Can you work these out from the model? Positions are in its coordinate system, mm. Face numbers are marked on the shaded views. A direction names the side the tool comes from. Round coordinates to 2 decimals unless told otherwise and drop trailing zeros. Loops run counter-clockwise (first coordinate to the right, second up) from the corner with the lowest first, then second, coordinate; pieces in that order, holes last. Notation, with made-up numbers: M 66.5,-24 L 88.5,-24 A23 ccw 88.5,14 Z; hole C -9.5,36.25 d4. An arc over 180 degrees is marked long. Answer as CSV lines item,"result".
from build123d import *

# Parameters (mm, degrees)
SKETCH1_R           = 2.75
BOSS_EXTRUDE1_DEPTH = 30
CUT_EXTRUDE1_DEPTH  = 27
SKETCH4_3_R         = 6
CUT_EXTRUDE2_DEPTH  = 27


with BuildPart() as part:
    # Sketch1 → Boss-Extrude1 (new body)
    with BuildSketch(Plane(origin=(0, 0, 0), x_dir=(1, 0, 0), z_dir=(0, 1, 0))):
        with BuildLine():
            Line((42, 10.085339835), (-42, 10.085339835))
            ThreePointArc((-42, 10.085339835), (-52.085339835, 0), (-42, -10.085339835))
            Line((-42, -10.085339835), (42, -10.085339835))
            ThreePointArc((42, -10.085339835), (52.085339835, 0), (42, 10.085339835))
        make_face()
        with Locations((-42, 0)):
            Circle(SKETCH1_R, mode=Mode.SUBTRACT)
        with Locations((42, 0)):
            Circle(SKETCH1_R, mode=Mode.SUBTRACT)
    extrude(amount=BOSS_EXTRUDE1_DEPTH)

    # Sketch4 → Cut-Extrude1 (cut)
    with BuildSketch(Plane(origin=(0, 0, -10.085339835), x_dir=(-1, 0, 0), z_dir=(0, 0, -1))):
        Polygon((42, 21), (42, 15), (42, 9), (67.854954683, 9), (67.854954683, 21), align=None)
        Polygon((42, 9), (42, 15), (42, 21), (27, 21), (27, 9), align=None)
        Polygon((-42, 15), (-42, 9), (-27, 9), (-27, 21), (-42, 21), align=None)
        Polygon((-67.854954683, 21), (-67.854954683, 9), (-42, 9), (-42, 15), (-42, 21), align=None)
    extrude(amount=-CUT_EXTRUDE1_DEPTH, mode=Mode.SUBTRACT)

    # Sketch4_3 → Cut-Extrude2 (cut)
    with BuildSketch(Plane(origin=(0, 0, -10.085339835), x_dir=(-1, 0, 0), z_dir=(0, 0, -1))):
        with Locations((0, 15)):
            Circle(SKETCH4_3_R)
    extrude(amount=-CUT_EXTRUDE2_DEPTH, mode=Mode.SUBTRACT)


solid = part.part
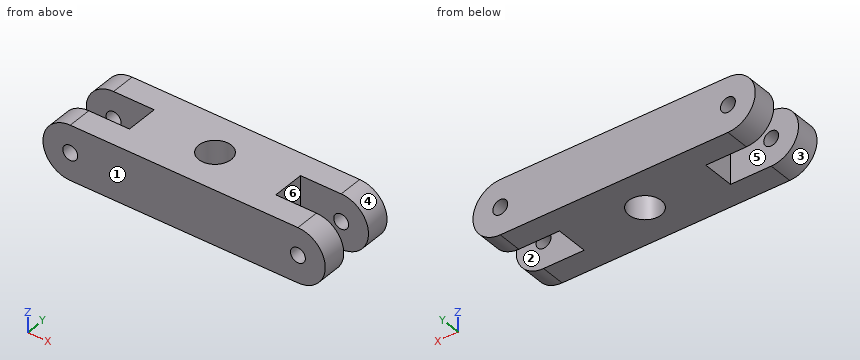
Item 1: On a 3-axis mill with a long thin cutter (end or side, diameter ignored), from which of +Z, -Z, +X, -X, +Y, -Y can I reach the whole of each face in a straight line? I mean the marked faces 4, 5 and 6. Say none if no direction works.
Output:
face 4,"+X, +Y, -Y"
face 5,"+Z, -Z, -X"
face 6,"+Z, -Z, +X"
Item 2: If we section it at B-B on x = 0: Write out the boundary of the cut face in (y, z), then the cut area to 3 significant figures.
Output:
outline,"M 0,-10.09 L 9,-10.09 L 9,10.09 L 0,10.09 Z; M 21,-10.09 L 30,-10.09 L 30,10.09 L 21,10.09 Z"
area,"363 mm2"
Item 3: If we section it at D-D on z = 6: Write out the boundary of the cut face in (x, y), then the cut area to 3 significant figures.
Output:
outline,"M -50.11,0 L 50.11,0 L 50.11,9 L 27,9 L 27,21 L 50.11,21 L 50.11,30 L -50.11,30 L -50.11,21 L -27,21 L -27,9 L -50.11,9 Z; hole C 0,15 d12"
area,"2,340 mm2"
Item 4: If I drill on line 1 along Y through (x, z) = (29, 9); line 2 along X through (y, z) = (4.75, 0); line 3 along X through (y, z) = (3, -1.75), over which ranges is the centre line in solid material (lowest first)? Write a range as from..to.
Output:
line 1,"y = 0..9, 21..30"
line 2,"x = -52.09..-44.75, -39.25..39.25, 44.75..52.09"
line 3,"x = -51.93..-44.12, -39.88..39.88, 44.12..51.93"
Item 5: Will these pins go through, and if not, where does the flat tip stop? pin 1 (6 mm diameter, centred on y = 15, z = 1.5, fed in from +X); pin 2 (5 mm diameter, centred on x = 42, z = 0, fed in from +Y); pin 3 (5 mm diameter, centred on y = 21.5, z = 7.5, fed in from +X); pin 4 (10 mm diameter, centred on y = 22.5, z = -6.5, fed in from +X).
Output:
pin 1,"stops at x = 27"
pin 2,"passes through"
pin 3,"stops at x = 50.76"
pin 4,"stops at x = 51.97"
Item 6: We'd pull the mould along Y, two halves only. Please class the marked faces 1, 2 and 3: released by +Y, released by -Y, zero draft, split by the parting line, or undercut.
Output:
face 1,"released by -Y"
face 2,"undercut"
face 3,"zero draft"
Item 7: If we section it at C-C on y = 15: Write out the boundary of the cut face in (x, z).
Output:
outline,"M -27,-10.09 L -6,-10.09 L -6,10.09 L -27,10.09 Z; M 6,-10.09 L 27,-10.09 L 27,10.09 L 6,10.09 Z"
Item 8: If we section it at A-A on z = 0: State how many separate pieces and enclosed holes the cut face has, then the cut area to 3 significant figures.
Output:
separate pieces,"5"
enclosed holes,"1"
area,"2,210 mm2"
